Design review of the part built by this model. Coordinates are the model's own, in mm. A direction names the side the tool comes from. Coordinates: 2 decimals unless noted, no trailing zeros. Write each loop counter-clockwise with the first axis right and the second up, starting at its lowest first coordinate (ties: lowest second). Pieces come first, ordered by that corner, then holes.
Q1. For probe 1 along X at (y, z) = (-2, 2.5); probe 2 along X at (y, z) = (0.5, 3.5); probe 3 along Z at (x, y) = (-9.5, 0.5), list the stretches that pass through material, from the lowest coordinate up.
Q2. Machinability: for faces 1 (the cylindrical face through (-32.5, 0.17, 0.05)), 2 (the flat face through (-12, -7.494, 0)), 3 (the flat face through (-12, 7.506, 0)), which of the approach directions +Z, -Z, +X, -X, +Y, -Y give a long, thin tool a straight path to every point of the face, cutting with its end or side? Answer none if there is none.
Q3. Take a section at B-B (y = 1.5). Give the boundary of the cut face in (x, z).
Q4. Take a section at C-C (y = -5). Give the boundary of the cut face in (x, z).
Q5. Take a section at D-D (x = -19). Give the boundary of the cut face in (y, z).
Q6. Take a section at A-A (z = 2). State how many separate pieces and enclosed holes the cut face has, and give its area (3 significant figures).
Q7. Insertion check: pin 1 (6 mm diameter, centred on x = -15.5, z = -0.5, fed in from +Y); pin 2 (4 mm diameter, centred on x = 23, y = 7, fed in from +Z); pin 3 (2 mm diameter, centred on y = -6.5, z = 4, fed in from +X). Each pin has a flat end and moves straight along its axis. Give the tip position at first contact, or say it passes through.
```python
from build123d import *

# Parameters (mm, degrees)
BOSS_EXTRUDE1_DEPTH = 3.75
SKETCH2_R           = 10
BOSS_EXTRUDE2_DEPTH = 5


with BuildPart() as part:
    # Sketch1 → Boss-Extrude1 (new, symmetric)
    with BuildSketch(Plane.XY):
        with BuildLine():
            ThreePointArc((-17.5, 0.005872539), (-19.696699141, 5.309173398), (-25, 7.505872539))
            Line((-25, 7.505872539), (-25, 2.505872539))
            ThreePointArc((-25, 2.505872539), (-23.232233047, 1.773639492), (-22.5, 0.005872539))
            Line((-22.5, 0.005872539), (-17.5, 0.005872539))
        make_face()
        with BuildLine():
            Line((-25, 2.505872539), (-25, 7.505872539))
            ThreePointArc((-25, 7.505872539), (-30.303300859, 5.309173398), (-32.5, 0.005872539))
            Line((-32.5, 0.005872539), (-27.5, 0.005872539))
            ThreePointArc((-27.5, 0.005872539), (-26.767766953, 1.773639492), (-25, 2.505872539))
        make_face()
        with BuildLine():
            ThreePointArc((-25, -7.494127461), (-19.696699141, -5.29742832), (-17.5, 0.005872539))
            Line((-17.5, 0.005872539), (-22.5, 0.005872539))
            ThreePointArc((-22.5, 0.005872539), (-23.232233047, -1.761894414), (-25, -2.494127461))
            Line((-25, -2.494127461), (-25, -7.494127461))
        make_face()
        with BuildLine():
            Line((-27.5, 0.005872539), (-32.5, 0.005872539))
            ThreePointArc((-32.5, 0.005872539), (-30.303300859, -5.29742832), (-25, -7.494127461))
            Line((-25, -7.494127461), (-25, -2.494127461))
            ThreePointArc((-25, -2.494127461), (-26.767766953, -1.761894414), (-27.5, 0.005872539))
        make_face()
        with BuildLine():
            ThreePointArc((50.201457579, -5.763117708), (54.152393819, -4.00404756), (55.772506702, 0.005872539))
            Line((55.772506702, 0.005872539), (2.499993103, 0.005872539))
            ThreePointArc((2.499993103, 0.005872539), (2.499998276, 0.002936272), (2.5, 0))
            ThreePointArc((2.5, 0), (1.869738707, -1.659541253), (0.296738265, -2.482326812))
            ThreePointArc((0.296738265, -2.482326812), (-1.661736132, -1.867788272), (-2.499993103, 0.005872539))
            Line((-2.499993103, 0.005872539), (-17.5, 0.005872539))
            ThreePointArc((-17.5, 0.005872539), (-19.696699141, -5.29742832), (-25, -7.494127461))
            Line((-25, -7.494127461), (0.631823856, -7.494127461))
            Line((0.631823856, -7.494127461), (50.201457579, -5.763117708))
        make_face()
        with BuildLine():
            Line((50.201457579, 5.774862786), (0.631823856, 7.505872539))
            Line((0.631823856, 7.505872539), (-25, 7.505872539))
            ThreePointArc((-25, 7.505872539), (-19.696699141, 5.309173398), (-17.5, 0.005872539))
            Line((-17.5, 0.005872539), (-2.499993103, 0.005872539))
            ThreePointArc((-2.499993103, 0.005872539), (-1.657344084, 1.871686562), (0.296738265, 2.482326812))
            ThreePointArc((0.296738265, 2.482326812), (1.867788272, 1.661736132), (2.499993103, 0.005872539))
            Line((2.499993103, 0.005872539), (55.772506702, 0.005872539))
            ThreePointArc((55.772506702, 0.005872539), (54.152393819, 4.015792638), (50.201457579, 5.774862786))
        make_face()
    extrude(amount=BOSS_EXTRUDE1_DEPTH, both=True)

    # Sketch2 → Boss-Extrude2 (add, symmetric)
    with BuildSketch(Plane.XY):
        with Locations((50.201457579, 0.005872539)):
            Circle(SKETCH2_R)
    extrude(amount=BOSS_EXTRUDE2_DEPTH, both=True)


solid = part.part
```
Response:
1. probe 1: x = -32.23 to -26.49, -23.51 to -1.5, 1.5 to 60
1. probe 2: x = -32.48 to -27.45, -22.55 to -2.45, 2.45 to 60.19
1. probe 3: z = -3.75 to 3.75
2. face 1: +Z, -Z, -X
2. face 2: +Z, -Z, -X, -Y
2. face 3: +Z, -Z, -X, +Y
3. outline: (-32.35, -3.75) - (-27, -3.75) - (-27, 3.75) - (-32.35, 3.75) - close; (-23, -3.75) - (-2, -3.75) - (-2, 3.75) - (-23, 3.75) - close; (2, -3.75) - (40.31, -3.75) - (40.31, -5) - (60.09, -5) - (60.09, 5) - (40.31, 5) - (40.31, 3.75) - (2, 3.75) - close
4. outline: (-30.58, -3.75) - (41.54, -3.75) - (41.54, -5) - (58.86, -5) - (58.86, 5) - (41.54, 5) - (41.54, 3.75) - (-30.58, 3.75) - close
5. outline: (-7.49, -3.75) - (7.51, -3.75) - (7.51, 3.75) - (-7.49, 3.75) - close
6. separate pieces: 1
6. enclosed holes: 2
6. area: 1,290 mm2
7. pin 1: stops at y = 7.51
7. pin 2: stops at z = 3.75
7. pin 3: stops at x = 58.55
